Check sheet for the modelled part. Datum: model origin and axes. Units: mm. A direction names the side the tool comes from. Round coordinates to 2 decimals unless told otherwise and drop trailing zeros. Write each loop counter-clockwise with the first axis right and the second up, starting at its lowest first coordinate (ties: lowest second). Pieces come first, ordered by that corner, then holes. Notation, with made-up numbers: (16.5, 60.25) -> (61.5, 60.25) arc R3 ccw to (61.5, 65.25) -> close; hole circle Ø1 at (54, -5.75). An arc over 180 degrees is marked (long way). One line per item, written item: value.
from build123d import *

# Parameters (mm, degrees)
SKETCH1_W           = 150
SKETCH1_H           = 150
BOSS_EXTRUDE1_DEPTH = 15
SKETCH2_W           = 20.0000108
SKETCH2_H           = 40.894
CUT_EXTRUDE1_DEPTH  = 15
SKETCH4_W           = 25
SKETCH4_H           = 25
BOSS_EXTRUDE2_DEPTH = 38.222
FILLET1_R           = 10
FILLET2_R           = 4
SKETCH5_R           = 2
SKETCH5_R_2         = 2.01
CUT_EXTRUDE2_DEPTH  = 53.222


with BuildPart() as part:
    # Sketch1 → Boss-Extrude1 (new body)
    with BuildSketch(Plane(origin=(0, 0, 0), x_dir=(1, 0, 0), z_dir=(0, 1, 0))):
        with Locations((-75, 75)):
            Rectangle(SKETCH1_W, SKETCH1_H)
    extrude(amount=BOSS_EXTRUDE1_DEPTH)

    # Sketch2 → Cut-Extrude1 (cut)
    with BuildSketch(Plane(origin=(0, 15, 0), x_dir=(1, 0, 0), z_dir=(0, 1, 0))):
        with Locations((-75, 75)):
            Rectangle(SKETCH2_W, SKETCH2_H)
    extrude(amount=-CUT_EXTRUDE1_DEPTH, mode=Mode.SUBTRACT)

    # Sketch4 → Boss-Extrude2 (add)
    with BuildSketch(Plane.XZ):
        with Locations((-137.5, -12.5)):
            Rectangle(SKETCH4_W, SKETCH4_H)
        with Locations((-137.5, -137.5)):
            Rectangle(SKETCH4_W, SKETCH4_H)
        with Locations((-12.5, -12.5)):
            Rectangle(SKETCH4_W, SKETCH4_H)
        with Locations((-12.5, -137.5)):
            Rectangle(SKETCH4_W, SKETCH4_H)
    extrude(amount=BOSS_EXTRUDE2_DEPTH)

    # Fillet1
    fillet1_edges = [part.edges().sort_by_distance(p)[0] for p in [
        (-75, 0, 0),
        (-137.5, 0, -25),
        (-150, -19.111, -25),
        (-125, 0, -12.5),
        (-125, -19.111, 0),
        (-150, 0, -75),
        (-125, 0, -137.5),
        (-125, -19.111, -150),
        (-137.5, 0, -125),
        (-150, -19.111, -125),
        (0, 0, -75),
        (-25, 0, -12.5),
        (-25, -19.111, 0),
        (-12.5, 0, -25),
        (0, -19.111, -25),
        (-75, 0, -150),
        (-12.5, 0, -125),
        (0, -19.111, -125),
        (-25, 0, -137.5),
        (-25, -19.111, -150),
    ]]
    fillet(fillet1_edges, radius=FILLET1_R)

    # Fillet2
    fillet2_edges = [part.edges().sort_by_distance(p)[0] for p in [
        (-150, 15, -75),
        (-75, 15, 0),
        (0, 15, -75),
        (0, -11.611, 0),
        (-150, -11.611, 0),
        (-150, -11.611, -150),
        (0, -11.611, -150),
        (-75, 15, -150),
    ]]
    fillet(fillet2_edges, radius=FILLET2_R)

    # Sketch5 → Cut-Extrude2 (cut)
    with BuildSketch(Plane(origin=(0, 15, 0), x_dir=(1, 0, 0), z_dir=(0, 1, 0))):
        with Locations(Location((-80, 50.25, 0), (0, 0, 270))):
            Circle(SKETCH5_R)
        with Locations(Location((-70, 50.25, 0), (0, 0, 270))):
            Circle(SKETCH5_R)
        with Locations(Location((-80, 99.75, 0), (0, 0, 270))):
            Circle(SKETCH5_R_2)
        with Locations(Location((-70, 99.75, 0), (0, 0, 270))):
            Circle(SKETCH5_R_2)
    extrude(amount=-CUT_EXTRUDE2_DEPTH, mode=Mode.SUBTRACT)


solid = part.part
Item 1: Sectioned sample at A-A (y = -22). Enter the section's corners in (x, z), then the cut area to 3 significant figures.
Result set:
outline: (-150, -146) arc R4 ccw to (-146, -150) -> (-135, -150) arc R10 ccw to (-125, -140) -> (-125, -125) -> (-140, -125) arc R10 ccw to (-150, -135) -> close; (-150, -15) arc R10 ccw to (-140, -25) -> (-125, -25) -> (-125, -10) arc R10 ccw to (-135, 0) -> (-146, 0) arc R4 ccw to (-150, -4) -> close; (-25, -140) arc R10 ccw to (-15, -150) -> (-4, -150) arc R4 ccw to (0, -146) -> (0, -135) arc R10 ccw to (-10, -125) -> (-25, -125) -> close; (-25, -25) -> (-10, -25) arc R10 ccw to (0, -15) -> (0, -4) arc R4 ccw to (-4, 0) -> (-15, 0) arc R10 ccw to (-25, -10) -> close
area: 2,310 mm^2
Item 2: Release check for a two-part mould opening along Z. For faces 6 (the cylindrical face through (-148.859, -13.266, -1.203)), 7 (the cylindrical face through (-78.017, 7.605, -50.51)), 8 (the flat face through (-123, 10, -150)), 9 (the flat face through (-125, -24, -18)) record: pulls with the +Z half, pulls with the -Z half, needs draft (parallel to the pull), parting line crosses it, or undercut.
Result set:
face 6: pulls with the +Z half
face 7: undercut
face 8: pulls with the -Z half
face 9: needs draft
Item 3: Sectioned sample at B-B (z = -50.25). Enter the section's corners in (x, y), then the cut area to 3 significant figures.
Result set:
outline: (-150, 10) arc R10 ccw to (-140, 0) -> (-82, 0) -> (-82, 15) -> (-146, 15) arc R4 ccw to (-150, 11) -> close; (-78, 0) -> (-72, 0) -> (-72, 15) -> (-78, 15) -> close; (-68, 0) -> (-10, 0) arc R10 ccw to (0, 10) -> (0, 11) arc R4 ccw to (-4, 15) -> (-68, 15) -> close
area: 2,080 mm^2
Item 4: Material ranges on line 1 along X through (y, z) = (-25.5, -135); line 2 along Y through (x, z) = (-86, -26.5); line 3 along X through (y, z) = (6.25, -50.25), recorded low to high.
Result set:
line 1: -150 to -125, -25 to 0
line 2: 0 to 15
line 3: -149.27 to -82, -78 to -72, -68 to -0.73
Item 5: Tool access check on faces 1 (the cylindrical face through (-147.15, -24.31, -128.01)), 2 (the flat face through (-90, 0, -76)), 3 (the cylindrical face through (-74.44, 2.85, -146.99)), 4 (the flat face through (-18, -24, -125)), 5 (the cylindrical face through (-28.01, -2.85, -130.1)). Record the directions out of +Z, -Z, +X, -X, +Y, -Y that give a thin tool (end or side, any length) a straight path to the whole face; none if there is none.
Result set:
face 1: -X, -Y
face 2: -Y
face 3: -Z, -Y
face 4: +X, -X, -Y
face 5: +Z, -Z, -Y
Item 6: Depth check by flat-ended pin: pin 1 (1.5 mm diameter, centred on x = -70.5, z = -35, fed in from -Y); pin 2 (1.5 mm diameter, centred on x = -20.5, y = -2, fed in from -Z); pin 3 (4.5 mm diameter, centred on x = -18.5, y = -21.5, fed in from -Z). Enter the tip coordinate at first touch or a pass-through.
Result set:
pin 1: y = 0
pin 2: z = -149.63
pin 3: z = -149.92
Item 7: Sectioned sample at D-D (z = -99.75). Enter the section's corners in (x, y).
Result set:
outline: (-150, 10) arc R10 ccw to (-140, 0) -> (-82.01, 0) -> (-82.01, 15) -> (-146, 15) arc R4 ccw to (-150, 11) -> close; (-77.99, 0) -> (-72.01, 0) -> (-72.01, 15) -> (-77.99, 15) -> close; (-67.99, 0) -> (-10, 0) arc R10 ccw to (0, 10) -> (0, 11) arc R4 ccw to (-4, 15) -> (-67.99, 15) -> close
Item 8: Sectioned sample at C-C (x = -80). Enter the section's corners in (y, z).
Result set:
outline: (0, -140) arc R10 ccw to (10, -150) -> (11, -150) arc R4 ccw to (15, -146) -> (15, -101.76) -> (0, -101.76) -> close; (0, -97.74) -> (15, -97.74) -> (15, -95.45) -> (0, -95.45) -> close; (0, -54.55) -> (15, -54.55) -> (15, -52.25) -> (0, -52.25) -> close; (0, -48.25) -> (15, -48.25) -> (15, -4) arc R4 ccw to (11, 0) -> (10, 0) arc R10 ccw to (0, -10) -> close
